```python
from build123d import *

# Parameters (mm, degrees)
VERTICAL_WALL_DEPTH           = 0.65
SMALL_END_ARM_DEPTH           = 75
SKETCH10_W                    = 13
SKETCH10_H                    = 35.229215797
SMALL_END_SLOTS_DEPTH         = 0.65
EDGE_FLANGE4_STRIP_W          = 4.0732
EDGE_FLANGE4_STRIP_H          = 0.65
EDGE_FLANGE4_STRIP_CUT_DEPTH  = 20
EDGE_FLANGE4_RELIEF_W         = 4.3982
EDGE_FLANGE4_RELIEF_H         = 0.325
EDGE_FLANGE4_RELIEF_CUT_DEPTH = 0.65
EDGE_FLANGE4_DEPTH            = 20
SKETCH28_R                    = 1.5
GUARD_MOUNTING_HOLES_2_DEPTH  = 0.65
CUT_EXTRUDE1_START            = -80
CUT_EXTRUDE1_DEPTH            = 35
M3_CLEARANCE_HOLE1_D          = 3.4
M3_CLEARANCE_HOLE1_DEPTH      = 10
M3_CLEARANCE_HOLE1_TIP        = 1.021463052


# Read off the part's stored shape, not the designer's step: Cut-Extrude1
# Sheet-metal steps are written as plain solids
with BuildPart() as part:
    # Sketch1 → Vertical Wall (new body)
    with BuildSketch(Plane(origin=(0, 0, 0), x_dir=(1, 0, 0), z_dir=(0, 1, 0))):
        Polygon((0, 0), (15, 0), (15, 80), (0.01, 75.000714286), (0, 75), align=None)
    extrude(amount=-VERTICAL_WALL_DEPTH)

    # Small End Arm section (across the edge) → Small End Arm (add)
    with BuildSketch(Plane(origin=(-0.682114537, 0, -75), x_dir=(0.9970544854948823, 0.07669649897182769, 0), z_dir=(0, 0, 1))):
        with BuildLine():
            Line((-0.65, 0.682114537), (-0.65, 75))
            Line((-0.65, 75), (0, 75))
            Line((0, 75), (0, 0.682114537))
            ThreePointArc((0, 0.682114537), (0.196140236, 0.181631966), (0.680105359, -0.052315797))
            Line((0.680105359, -0.052315797), (0.630252635, -0.700401212))
            ThreePointArc((0.630252635, -0.700401212), (-0.280779186, -0.26001027), (-0.65, 0.682114537))
        make_face()
    extrude(amount=SMALL_END_ARM_DEPTH)

    # Sketch10 → Small End Slots (cut)
    with BuildSketch(Plane(origin=(-1.326187514, -0.102014424, 0), x_dir=(0, 0, 1), z_dir=(-0.9970544854948824, -0.07669649897182769, 0))):
        with Locations((-25.9123, 57.437707899)):
            Rectangle(SKETCH10_W, SKETCH10_H)
        with BuildLine():
            Line((-39.4123, 75.052315797), (-39.4123, 39.770784203))
            ThreePointArc((-39.4123, 39.770784203), (-40.9123, 38.270784203), (-42.4123, 39.770784203))
            Line((-42.4123, 39.770784203), (-42.4123, 75.052315797))
            ThreePointArc((-42.4123, 75.052315797), (-40.9123, 76.552315797), (-39.4123, 75.052315797))
        make_face()
        with BuildLine():
            Line((-9.4123, 75.052315797), (-9.4123, 39.770784203))
            ThreePointArc((-9.4123, 39.770784203), (-10.9123, 38.270784203), (-12.4123, 39.770784203))
            Line((-12.4123, 39.770784203), (-12.4123, 75.052315797))
            ThreePointArc((-12.4123, 75.052315797), (-10.9123, 76.552315797), (-9.4123, 75.052315797))
        make_face()
    extrude(amount=-SMALL_END_SLOTS_DEPTH, mode=Mode.SUBTRACT)

    # Edge-Flange4 strip (across the edge) → Edge-Flange4 strip cut (cut)
    with BuildSketch(Plane(origin=(-5.548507396, 54.788143978, 0), x_dir=(0, 0, -1), z_dir=(-0.0766964989718277, 0.9970544854948823, 0))):
        with Locations((-0.65, -0.325)):
            Rectangle(EDGE_FLANGE4_STRIP_W, EDGE_FLANGE4_STRIP_H)
    extrude(amount=EDGE_FLANGE4_STRIP_CUT_DEPTH, mode=Mode.SUBTRACT)

    # Edge-Flange4 relief (on the sheet) → Edge-Flange4 relief cut (cut)
    with BuildSketch(Plane(origin=(-5.548507396, 54.788143978, -1.3866), x_dir=(0, 0, -1), z_dir=(-0.9970544854948823, -0.0766964989718277, 6.982374222178593e-15))):
        with Locations((-1.8741, 0.1625)):
            Rectangle(EDGE_FLANGE4_RELIEF_W, EDGE_FLANGE4_RELIEF_H)
    extrude(amount=-EDGE_FLANGE4_RELIEF_CUT_DEPTH, mode=Mode.SUBTRACT)

    # Edge-Flange4 section (across the edge) → Edge-Flange4 (add)
    with BuildSketch(Plane(origin=(-5.548507396, 54.788143978, 0), x_dir=(0, 0, -1), z_dir=(-0.0766964989718277, 0.9970544854948823, 0))):
        with BuildLine():
            Line((0, 0.7366), (0, 10))
            Line((0, 10), (0.65, 10))
            Line((0.65, 10), (0.65, 0.7366))
            ThreePointArc((0.65, 0.7366), (0.865745145, 0.215745145), (1.3866, 0))
            Line((1.3866, 0), (1.3866, -0.65))
            ThreePointArc((1.3866, -0.65), (0.406125737, -0.243874263), (0, 0.7366))
        make_face()
    extrude(amount=EDGE_FLANGE4_DEPTH)

    # Sketch28 → Guard Mounting Holes 2 (cut)
    with BuildSketch(Plane(origin=(-1.326187514, -0.102014424, 0), x_dir=(0, 0, 1), z_dir=(-0.9970544854948823, -0.07669649897182768, 0))):
        with Locations(Location((-68.282596145, 53.577296087, 0), (0, 0, 270))):
            Circle(SKETCH28_R)
        with Locations(Location((-68.282596145, 41.577296087, 0), (0, 0, 270))):
            Circle(SKETCH28_R)
    extrude(amount=-GUARD_MOUNTING_HOLES_2_DEPTH, mode=Mode.SUBTRACT)

    # Cut-Extrude1 outline → Cut-Extrude1 (cut)
    with BuildSketch(Plane.XY.offset(CUT_EXTRUDE1_START)):
        with BuildLine():
            Line((-0.734430334, 0.680105359), (-1.38251575, 0.630252635))
            ThreePointArc((-1.38251575, 0.630252635), (-0.942124807, -0.280779186), (0, -0.65))
            Line((0, -0.65), (15, -0.65))
            Line((15, -0.65), (15, 0))
            Line((15, 0), (0, 0))
            ThreePointArc((0, 0), (-0.500482571, 0.196140236), (-0.734430334, 0.680105359))
        make_face()
    extrude(amount=CUT_EXTRUDE1_DEPTH, mode=Mode.SUBTRACT)

    # M3 Clearance Hole1
    with Locations(Plane(origin=(0, 0, -0.65), x_dir=(-1, 0, 0), z_dir=(0, 0, -1))):
        with Locations((11.300744813, 64.375206338)):
            Hole(M3_CLEARANCE_HOLE1_D / 2, depth=M3_CLEARANCE_HOLE1_DEPTH)
            with Locations((0, 0, -(M3_CLEARANCE_HOLE1_DEPTH + M3_CLEARANCE_HOLE1_TIP / 2))):  # 118° drill point
                Cone(0, M3_CLEARANCE_HOLE1_D / 2, M3_CLEARANCE_HOLE1_TIP, mode=Mode.SUBTRACT)


solid = part.part
```
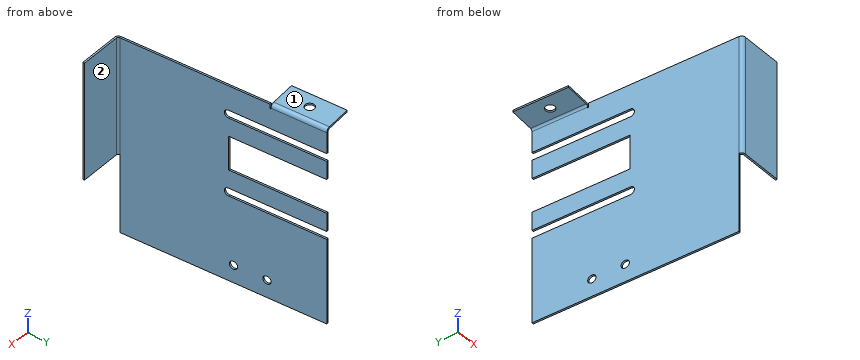
Design review of the part built by this model. Coordinates are the model's own, in mm. Face numbers are marked on the shaded views. A direction names the side the tool comes from. Give positions to 0.01 mm unless a question says otherwise; leave off trailing zeros. Loops run counter-clockwise (first coordinate to the right, second up) from the corner with the lowest first, then second, coordinate; pieces in that order, holes last. Notation, with made-up numbers: M 22,70.25 L 66,70.25 A14 cw 66,75.25 Z; hole C -23,12.5 d8. An arc over 180 degrees is marked long. Return JSON: item names as keys, results as strings. Group by question number.
Item 1: Tool access review of the marked faces 1 and 2: name each direction out of +Z, -Z, +X, -X, +Y, -Y from which nothing blocks a thin tool from reaching the whole face with its end or side.
Item 2: We need section A-A (z = -17). Give the boundary of the cut face in (x, y), and give its area (3 significant figures).
Item 3: We need section B-B (y = 48). Give the boundary of the cut face in (x, z), and give its area (3 significant figures).
Item 4: We need section C-C (x = -11.5). Give the boundary of the cut face in (y, z).
Item 5: For probe 1 along Z at (x, y) = (-11, 61); probe 2 along X at (y, z) = (67.5, -50.5), list the stretches that pass through material, from the lowest coordinate up.
Item 6: Insertion check: pin 1 Ø5.5 at (x, y) = (-11.3, 64.38) entering from +Z; pin 2 Ø5 at (y, z) = (28.5, -28) entering from -X; pin 3 Ø12 at (x, z) = (5.5, -30.5) entering from +Y; pin 4 Ø10 at (x, z) = (8.5, -29.5) entering from +Y. Each pin has a flat end and moves straight along its axis. Give the tip position at first contact, or say it passes through.
Item 7: We need section D-D (x = 4). Give the boundary of the cut face in (y, z), and give its area (4 significant figures).
Output:
{
 "1": {"face 1": "+Z, +X, -X, +Y, -Y", "face 2": "+Z, -Z, +X, +Y"},
 "2": {"outline": "M -7.08,74.73 L -1.38,0.63 A1.39 ccw 0,-0.65 L 15,-0.65 L 15,0 L 0,0 A0.74 cw -0.73,0.68 L -6.43,74.78 Z", "area": "59.1 mm^2"},
 "3": {"outline": "M -5.03,-75 L -4.37,-75 L -4.37,-42.41 L -5.03,-42.41 Z; M -5.03,-39.41 L -4.37,-39.41 L -4.37,-32.41 L -5.03,-32.41 Z; M -5.03,-19.41 L -4.37,-19.41 L -4.37,-12.41 L -5.03,-12.41 Z; M -5.03,-9.41 L -4.37,-9.41 L -4.37,0 L -5.03,0 Z", "area": "36.5 mm^2"},
 "4": {"outline": "M 54.33,-0.65 L 62.69,-0.65 L 62.69,0 L 54.33,0 Z; M 66.06,-0.65 L 74.39,-0.65 L 74.39,0 L 66.06,0 Z"},
 "5": {"probe 1": "z = -0.65 to 0", "probe 2": "x = -6.53 to -5.87"},
 "6": {"pin 1": "stops at z = 0", "pin 2": "stops at x = -3.72", "pin 3": "stops at y = 0.2", "pin 4": "stops at y = 0"},
 "7": {"outline": "M -0.65,-45 L 0,-45 L 0,0 L -0.65,0 Z", "area": "29.25 mm^2"}
}
